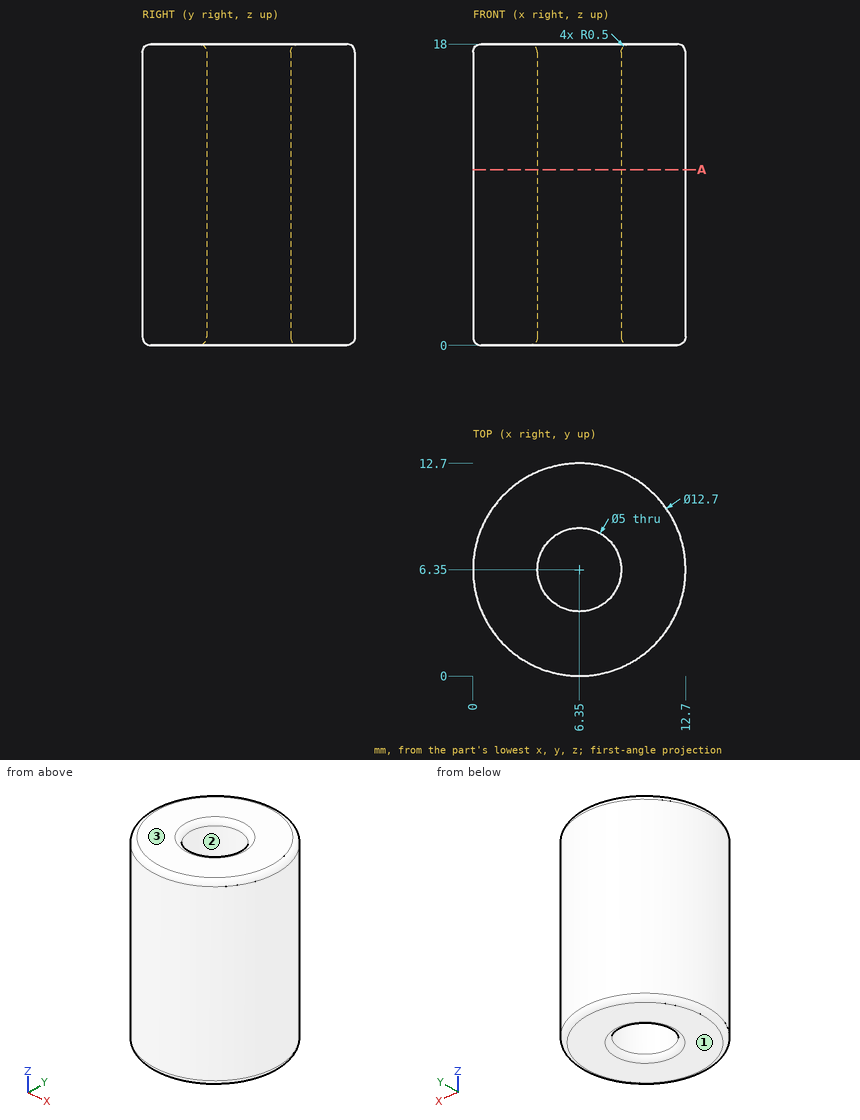
Design review of the part shown in the three views and the two pictorial views. Dimensions are in mm from the part's minimum x, y and z. Round coordinates to 2 decimals unless told otherwise and drop trailing zeros. Order: outer loops, then holes, each group sorted by start corner. A loop starts at its lowest first (then second) coordinate and runs counter-clockwise, first axis right, second up.
Q1. Insertion check: P1, Ø4, axis at x = 3, z = 12, coming from the -Y side; P2, Ø2, axis at y = 3, z = 10, coming from the -X side; P3, Ø1, axis at y = 7.5, z = 5, coming from the +X side. Each pin has a flat end and moves straight along its axis. Give the tip position at first contact, or say it passes through.
Findings below:
P1: stops at y = 0.15
P2: stops at x = 0.45
P3: stops at x = 12.67
Q2. Wall thickness on line 1 (X direction, y = 6.5, z = 5.5); line 2 (X direction, y = 7.5, z = 13.5) (3 decimals): over which ranges is each line inside the solid? List them lowest first.
Findings below:
line 1: x = 0 to 3.85, 8.85 to 12.7
line 2: x = 0.105 to 4.13, 8.57 to 12.595
Q3. We need section A-A, the plane z = 10.5. Give the boundary of the cut face in (x, y).
Findings below:
outline: circle Ø12.7 at (6.35, 6.35); hole circle Ø5 at (6.35, 6.35)
Q4. Mouldability with a two-part tool opening along Z and no side actions: class the marked faces 1, 2 and 3 as pulls with the +Z half, pulls with the -Z half, needs draft (parallel to the pull), parting line crosses it, or undercut.
Findings below:
face 1: pulls with the -Z half
face 2: needs draft
face 3: pulls with the +Z half
